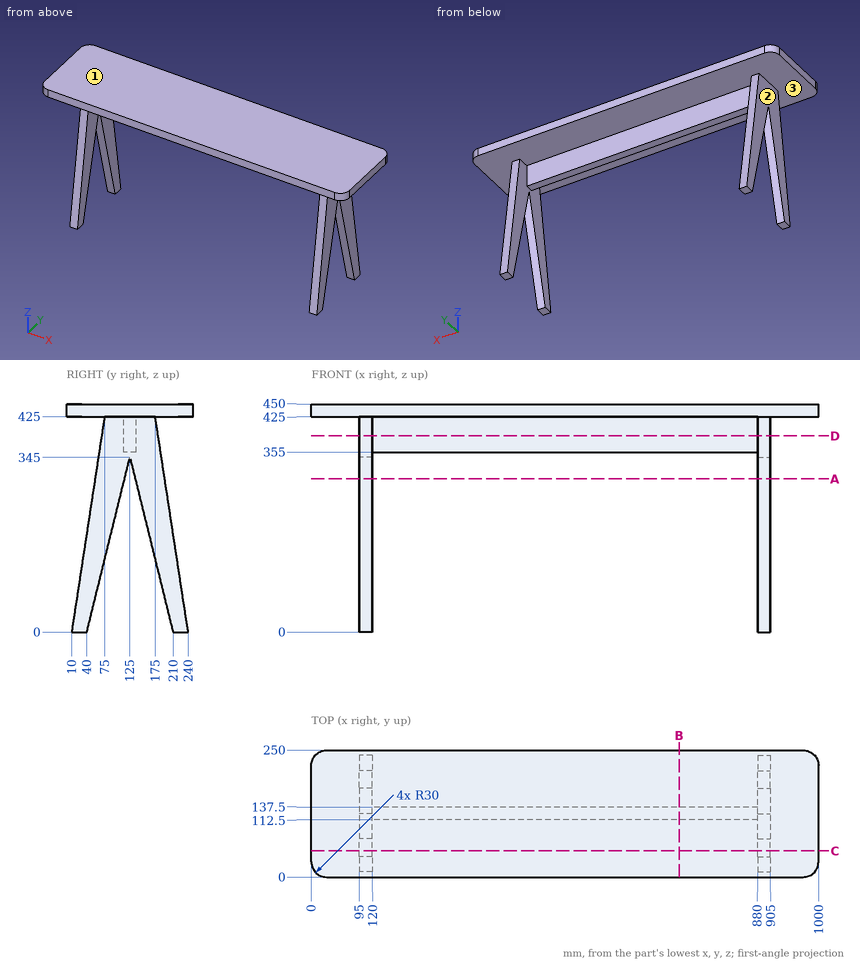
Study the drawing (mm; zero at the part's minimum x, y, z) and answer. Round coordinates to 2 decimals unless told otherwise and drop trailing zeros. Order: outer loops, then holes, each group sorted by start corner. A loop starts at its lowest first (then second) coordinate and runs counter-clockwise, first axis right, second up. Notation, with made-up numbers: (24, -17) -> (51, -17) arc R14 ccw to (51, 3) -> close; hole circle Ø5 at (7.5, 69). An arc over 180 degrees is marked (long way). Write each question's results on one line, items separated by ' | '. Start each with the question number.
Q1. Find section D-D (z = 387). Determine the outline of the cut face in (x, y).
Q2. The mould has two halves that part along X. Classify the marked faces 1, 2 and 3: pulls with the +X half, pulls with the -X half, needs draft (parallel to the pull), parting line crosses it, or undercut.
Q3. Straight lines are drawn through the part: probe 1 along X at (y, z) = (170, 210); probe 2 along Z at (x, y) = (348.5, 141.5); probe 3 along Y at (x, z) = (575, 379). For each, find the intervals that lie inside material, in ascending order. Write a range as from..to.
Q4. Find section C-C (y = 51.5). Determine the outline of the cut face in (x, z).
Q5. Find section B-B (x = 725). Determine the outline of the cut face in (y, z), then the cut area to 3 significant figures.
Q6. Find section A-A (z = 302.5). Determine the outline of the cut face in (x, y).
Q7. Each of these flat-tipped pins is pushed along its axis until it touches: pin 1 (10 mm diameter, centred on y = 60, z = 102, fed in from +X); pin 2 (8 mm diameter, centred on x = 572.5, y = 59, fed in from -Z). Where does it stop, or does it pass through?
Worked answers:
1) outline: (95, 69.19) -> (120, 69.19) -> (120, 112.5) -> (880, 112.5) -> (880, 69.19) -> (905, 69.19) -> (905, 180.81) -> (880, 180.81) -> (880, 137.5) -> (120, 137.5) -> (120, 180.81) -> (95, 180.81) -> close
2) face 1: needs draft | face 2: pulls with the -X half | face 3: undercut
3) probe 1: x = 95..120, 880..905 | probe 2: z = 425..450 | probe 3: y = 112.5..137.5
4) outline: (0, 425) -> (1000, 425) -> (1000, 450) -> (0, 450) -> close; (95, 46.68) -> (120, 46.68) -> (120, 271.35) -> (95, 271.35) -> close; (880, 46.68) -> (905, 46.68) -> (905, 271.35) -> (880, 271.35) -> close
5) outline: (0, 425) -> (112.5, 425) -> (112.5, 355) -> (137.5, 355) -> (137.5, 425) -> (250, 425) -> (250, 450) -> (0, 450) -> close | area: 8,000 mm2
6) outline: (95, 56.26) -> (120, 56.26) -> (120, 114.53) -> (95, 114.53) -> close; (95, 135.47) -> (120, 135.47) -> (120, 193.74) -> (95, 193.74) -> close; (880, 56.26) -> (905, 56.26) -> (905, 114.53) -> (880, 114.53) -> close; (880, 135.47) -> (905, 135.47) -> (905, 193.74) -> (880, 193.74) -> close
7) pin 1: stops at x = 905 | pin 2: stops at z = 425
